The model under review builds one solid part; all positions refer to its coordinate system, in mm. Round coordinates to 2 decimals unless told otherwise and drop trailing zeros. Order: outer loops, then holes, each group sorted by start corner. A loop starts at its lowest first (then second) coordinate and runs counter-clockwise, first axis right, second up.
```python
from build123d import *

# Parameters (mm, degrees)
F0_W          = 3.175
F0_H          = 4.7625
F1_DEPTH      = 7.1628
F2_R          = 2.286
F3_R          = 1.19126
F4_DEPTH      = 3.175
F5_R          = 0.79375
F6_DEPTH      = 25.4
F6_DEPTH_BACK = 25.4
F7_R          = 0.254


with BuildPart() as f1:
    # F0 (on Front) → F1 (new body)
    with BuildSketch(Plane.XZ):
        Rectangle(F0_W, F0_H)
    extrude(amount=F1_DEPTH)

    # F2
    f2_edges = [f1.edges().sort_by_distance(p)[0] for p in [
        (0, -7.1628, 2.38125),
        (0, -7.1628, -2.38125),
    ]]
    fillet(f2_edges, radius=F2_R)

    # F3 (on Front) → F4 (cut)
    with BuildSketch(Plane.XZ):
        Circle(F3_R)
    extrude(amount=F4_DEPTH, mode=Mode.SUBTRACT)

    # F5 (on Right) → F6 (cut, two sides)
    with BuildSketch(Plane.YZ) as f6_sk:
        with Locations((-4.7625, 0)):
            Circle(F5_R)
    extrude(amount=-F6_DEPTH, mode=Mode.SUBTRACT)
    extrude(f6_sk.sketch, amount=F6_DEPTH_BACK, mode=Mode.SUBTRACT)

    # F7
    f7_edges = [f1.edges().sort_by_distance(p)[0] for p in [
        (1.5875, -2.4384, 2.38125),
        (1.5875, -6.493246, 1.711696),
        (-1.5875, -6.493246, 1.711696),
        (-1.5875, -6.493246, -1.711696),
    ]]
    fillet(f7_edges, radius=F7_R)


solid = f1.part
```
(1) Draft analysis for pull direction X (two halves, no side actions). For faces 1 (the cylindrical face through (0.019, -6.475, 1.729)), 2 (the cylindrical face through (0.64, -1.565, 1.004)), 3 (the flat face through (1.588, -3, 0)), 4 (the flat face through (0, -3.175, 0)), state which applies: pulls with the +X half, pulls with the -X half, needs draft (parallel to the pull), parting line crosses it, or undercut.
Data:
face 1: needs draft
face 2: undercut
face 3: pulls with the +X half
face 4: undercut
(2) Consider section C-C (y = -1.75). Write out the cut boundary in (x, z), and give its area (3 significant figures).
Data:
outline: (-1.59, -2.13) arc R0.25 ccw to (-1.33, -2.38) - (1.33, -2.38) arc R0.25 ccw to (1.59, -2.13) - (1.59, 2.13) arc R0.25 ccw to (1.33, 2.38) - (-1.33, 2.38) arc R0.25 ccw to (-1.59, 2.13) - close; hole circle Ø2.38 at (0, 0)
area: 10.6 mm2
(3) To check wall thickness, follow probe 1 along Z at (x, y) = (0, -1.95); probe 2 along Y at (x, z) = (-0.85, 0) (3 decimals); probe 3 along Z at (x, y) = (-0.75, -4.75). State the ranges of each line that lie inside material, in increasing order.
Data:
probe 1: z = -2.38 to -1.19, 1.19 to 2.38
probe 2: y = -7.163 to -5.556, -3.969 to -3.175
probe 3: z = -2.38 to -0.79, 0.79 to 2.38
(4) Insertion check: pin 1 (0.7 mm diameter, centred on x = -0.5, z = 0.5, fed in from +Y) (3 decimals); pin 2 (1 mm diameter, centred on x = 1, z = 0.5, fed in from -Y); pin 3 (1.5 mm diameter, centred on x = -0.5, z = 2, fed in from -Y). Each pin has a flat end and moves straight along its axis. Give the tip position at first contact, or say it passes through.
Data:
pin 1: stops at y = -3.175
pin 2: stops at y = -7.16
pin 3: stops at y = -6.85
